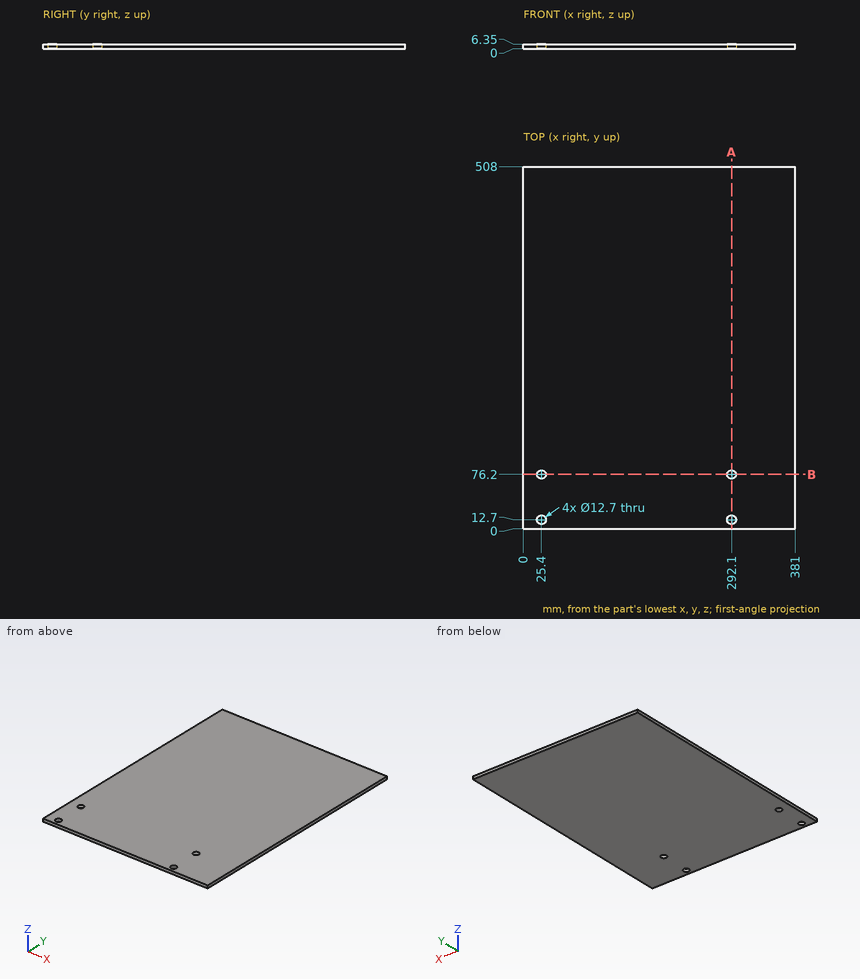
Geometry check sheet. Reference: drawing and pictorial views, mm from the part's lowest x, y, z. Round coordinates to 2 decimals unless told otherwise and drop trailing zeros. Loops run counter-clockwise (first coordinate to the right, second up) from the corner with the lowest first, then second, coordinate; pieces in that order, holes last.
1. Scan lines: probe 1 along Y at (x, z) = (25.4, 4); probe 2 along X at (y, z) = (77, 3.25). Record each from-to range of solid material in increasing order.
2. Sectioned sample at B-B on y = 76.2. Record the boundary of the cut face in (x, z), and give its area (3 significant figures).
3. Sectioned sample at A-A on x = 292.1. Record the boundary of the cut face in (y, z).
4. Gauge pin test, flat end, axial feed: pin 1 Ø7.5 at (x, y) = (292.1, 76.2) entering from -Z. Record the tip position at first contact, or that the pin passes through.
Recorded:
1. probe 1: y = 0 to 6.35, 19.05 to 69.85, 82.55 to 508
1. probe 2: x = 0 to 19.1, 31.7 to 285.8, 298.4 to 381
2. outline: (0, 0) - (19.05, 0) - (19.05, 6.35) - (0, 6.35) - close; (31.75, 0) - (285.75, 0) - (285.75, 6.35) - (31.75, 6.35) - close; (298.45, 0) - (381, 0) - (381, 6.35) - (298.45, 6.35) - close
2. area: 2,260 mm2
3. outline: (0, 0) - (6.35, 0) - (6.35, 6.35) - (0, 6.35) - close; (19.05, 0) - (69.85, 0) - (69.85, 6.35) - (19.05, 6.35) - close; (82.55, 0) - (508, 0) - (508, 6.35) - (82.55, 6.35) - close
4. pin 1: passes through
